For this review, take the finished solid that the model builds, in its own axes (mm). A direction names the side the tool comes from. Coordinates: 2 decimals unless noted, no trailing zeros. Write each loop counter-clockwise with the first axis right and the second up, starting at its lowest first coordinate (ties: lowest second). Pieces come first, ordered by that corner, then holes.
```python
from build123d import *

# Parameters (mm, degrees)
SKETCH2_R           = 2.0828
SKETCH2_W           = 57.15
SKETCH2_H           = 19.05
BOSS_EXTRUDE1_DEPTH = 3.175


with BuildPart() as part:
    # Sketch2 → Boss-Extrude1 (new body)
    with BuildSketch(Plane(origin=(0, 0, 0), x_dir=(1, 0, 0), z_dir=(0, 1, 0))):
        with BuildLine():
            Line((3.175, 0), (3.175, 12.7))
            Line((3.175, 12.7), (0, 12.7))
            Line((0, 12.7), (0, 25.4))
            Line((0, 25.4), (3.175, 25.4))
            Line((3.175, 25.4), (3.175, 38.1))
            Line((3.175, 38.1), (0, 38.1))
            Line((0, 38.1), (0, 50.8))
            Line((0, 50.8), (3.175, 50.8))
            Line((3.175, 50.8), (3.175, 63.5))
            Line((3.175, 63.5), (0, 63.5))
            Line((0, 63.5), (0, 76.2))
            Line((0, 76.2), (3.175, 76.2))
            Line((3.175, 76.2), (3.175, 88.9))
            Line((3.175, 88.9), (0, 88.9))
            Line((0, 88.9), (0, 101.6))
            Line((0, 101.6), (3.175, 101.6))
            Line((3.175, 101.6), (38.735, 101.6))
            ThreePointArc((38.735, 101.6), (41.275, 99.06), (43.815, 101.6))
            Line((43.815, 101.6), (102.235, 101.6))
            ThreePointArc((102.235, 101.6), (104.775, 99.06), (107.315, 101.6))
            Line((107.315, 101.6), (142.875, 101.6))
            Line((142.875, 101.6), (146.05, 101.6))
            Line((146.05, 101.6), (146.05, 88.9))
            Line((146.05, 88.9), (142.875, 88.9))
            Line((142.875, 88.9), (142.875, 76.2))
            Line((142.875, 76.2), (146.05, 76.2))
            Line((146.05, 76.2), (146.05, 63.5))
            Line((146.05, 63.5), (142.875, 63.5))
            Line((142.875, 63.5), (142.875, 50.8))
            Line((142.875, 50.8), (146.05, 50.8))
            Line((146.05, 50.8), (146.05, 38.1))
            Line((146.05, 38.1), (142.875, 38.1))
            Line((142.875, 38.1), (142.875, 25.4))
            Line((142.875, 25.4), (146.05, 25.4))
            Line((146.05, 25.4), (146.05, 12.7))
            Line((146.05, 12.7), (142.875, 12.7))
            Line((142.875, 12.7), (142.875, 0))
            Line((142.875, 0), (3.175, 0))
        make_face()
        with Locations(Location((136.525, 57.15, 0), (0, 0, 90))):
            Circle(SKETCH2_R, mode=Mode.SUBTRACT)
        with Locations(Location((9.525, 12.7, 0), (0, 0, 270))):
            Circle(SKETCH2_R, mode=Mode.SUBTRACT)
        with Locations(Location((9.525, 57.15, 0), (0, 0, 270))):
            Circle(SKETCH2_R, mode=Mode.SUBTRACT)
        with Locations(Location((136.525, 12.7, 0), (0, 0, 90))):
            Circle(SKETCH2_R, mode=Mode.SUBTRACT)
        with Locations(Location((28.575, 95.25, 0), (0, 0, 270))):
            Circle(SKETCH2_R, mode=Mode.SUBTRACT)
        with Locations(Location((117.475, 95.25, 0), (0, 0, 90))):
            Circle(SKETCH2_R, mode=Mode.SUBTRACT)
        with Locations(Location((66.675, 12.7, 0), (0, 0, 270))):
            Circle(SKETCH2_R, mode=Mode.SUBTRACT)
        with Locations(Location((79.375, 12.7, 0), (0, 0, 90))):
            Circle(SKETCH2_R, mode=Mode.SUBTRACT)
        with Locations((44.45, 60.325)):
            Rectangle(SKETCH2_W, SKETCH2_H, mode=Mode.SUBTRACT)
    extrude(amount=BOSS_EXTRUDE1_DEPTH)


solid = part.part
```
1) For L1, parallel to X at y = 2, z = -95.25; L2, parallel to X at y = 0.8, z = -57.15 (3 decimals); L3, parallel to Z at x = 69, y = 1.6, list the stretches that pass through material, from the lowest coordinate up.
2) Consider section C-C (z = -95.25). Give the boundary of the cut face in (x, y) (3 decimals), then the cut area to 3 significant figures.
3) Clearance check with flat-ended pins moving along their axes: P1, Ø1, axis at x = 1.5, y = 2, coming from the +Z side; P2, Ø1, axis at y = 2.5, z = -57.5, coming from the -X side (3 decimals); P3, Ø1.6, axis at y = 1, z = -56, coming from the +X side (3 decimals). State where each tip first meets the part, or that it passes through.
4) Consider section B-B (z = -57.15). Give the boundary of the cut face in (x, y) (3 decimals), then the cut area to 3 significant figures.
5) Consider section A-A (x = 50). Give the boundary of the cut face in (y, z) (3 decimals).
6) Consider section D-D (y = 0.8). Count the separate pieces of the cut face and the enclosed holes in it, then the cut area to 3 significant figures.
7) Tool access review of faces 4 (the face through (0, 2, -95)), 5 (the face through (3.175, 2, -82)), 6 (the face through (142.875, 2, -57)), 7 (the face through (73.025, 2, -60)): name each direction out of +Z, -Z, +X, -X, +Y, -Y from which nothing blocks a thin tool from reaching the whole face with its end or side.
8) The part is to be moulded in two halves that separate along X. For faces 1 (the face through (142.875, 2, -83)), 2 (the face through (3.175, 2, -32)), 3 (the face through (27.777, 1.565, -93.326)), say which applies: pulls with the +X half, pulls with the -X half, needs draft (parallel to the pull), parting line crosses it, or undercut.
Results:
1. L1: x = 0 to 26.49, 30.66 to 115.39, 119.56 to 146.05
1. L2: x = 3.175 to 7.442, 11.608 to 15.875, 73.025 to 134.442, 138.608 to 142.875
1. L3: z = -101.6 to -69.85, -50.8 to 0
2. outline: (0, 0) - (26.492, 0) - (26.492, 3.175) - (0, 3.175) - close; (30.658, 0) - (115.392, 0) - (115.392, 3.175) - (30.658, 3.175) - close; (119.558, 0) - (146.05, 0) - (146.05, 3.175) - (119.558, 3.175) - close
2. area: 437 mm2
3. P1: stops at z = -12.7
3. P2: stops at x = 3.175
3. P3: stops at x = 142.875
4. outline: (3.175, 0) - (7.442, 0) - (7.442, 3.175) - (3.175, 3.175) - close; (11.608, 0) - (15.875, 0) - (15.875, 3.175) - (11.608, 3.175) - close; (73.025, 0) - (134.442, 0) - (134.442, 3.175) - (73.025, 3.175) - close; (138.608, 0) - (142.875, 0) - (142.875, 3.175) - (138.608, 3.175) - close
4. area: 236 mm2
5. outline: (0, -101.6) - (3.175, -101.6) - (3.175, -69.85) - (0, -69.85) - close; (0, -50.8) - (3.175, -50.8) - (3.175, 0) - (0, 0) - close
6. separate pieces: 1
6. enclosed holes: 9
6. area: 13,300 mm2
7. face 4: +Z, -Z, -X, +Y, -Y
7. face 5: -X, +Y, -Y
7. face 6: +X, +Y, -Y
7. face 7: +Y, -Y
8. face 1: pulls with the +X half
8. face 2: pulls with the -X half
8. face 3: undercut
